```python
from build123d import *

# Parameters (mm, degrees)
SKETCH1_W           = 30.30738701
SKETCH1_H           = 30.002560534
BOSS_EXTRUDE1_DEPTH = 10
SKETCH2_R           = 9.6
SKETCH2_R_2         = 9.55
CUT_EXTRUDE1_DEPTH  = 7
SKETCH3_R           = 4
CUT_EXTRUDE2_DEPTH  = 10
SKETCH4_R           = 2
CUT_EXTRUDE3_DEPTH  = 10
CIRPATTERN1_COUNT   = 4


with BuildPart() as part:
    # Sketch1 → Boss-Extrude1 (new body)
    with BuildSketch(Plane(origin=(0, 0, 0), x_dir=(1, 0, 0), z_dir=(0, 1, 0))):
        Rectangle(SKETCH1_W, SKETCH1_H)
    extrude(amount=BOSS_EXTRUDE1_DEPTH)

    # Sketch2 → Cut-Extrude1 (cut)
    with BuildSketch(Plane(origin=(0, 10, 0), x_dir=(1, 0, 0), z_dir=(0, 1, 0))):
        Circle(SKETCH2_R)
        Circle(SKETCH2_R_2, mode=Mode.SUBTRACT)
    extrude(amount=-CUT_EXTRUDE1_DEPTH, mode=Mode.SUBTRACT)

    # Sketch3 → Cut-Extrude2 (cut)
    with BuildSketch(Plane(origin=(0, 10, 0), x_dir=(1, 0, 0), z_dir=(0, 1, 0))):
        Circle(SKETCH3_R)
    extrude(amount=-CUT_EXTRUDE2_DEPTH, mode=Mode.SUBTRACT)

    # Sketch4 → Cut-Extrude3 (cut)
    with BuildSketch(Plane(origin=(0, 10, 0), x_dir=(1, 0, 0), z_dir=(0, 1, 0))):
        with Locations((10.792349727, 10.987509758)):
            Circle(SKETCH4_R)
    cut_extrude3 = extrude(amount=-CUT_EXTRUDE3_DEPTH, mode=Mode.SUBTRACT)

    # CirPattern1: Cut-Extrude3 ×4 about axis
    cirpattern1_axis = Axis((0, 0, 0), (0, 1, 0))
    for i in range(1, CIRPATTERN1_COUNT):
        add(cut_extrude3.rotate(cirpattern1_axis, i * 360 / CIRPATTERN1_COUNT), mode=Mode.SUBTRACT)


solid = part.part
```
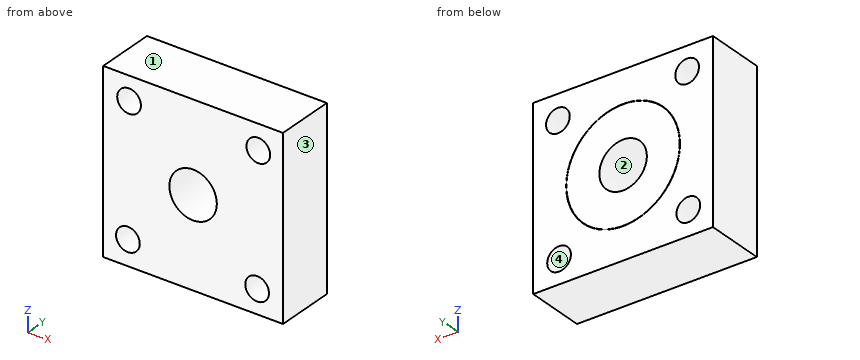
Read the model definition and answer for the solid it produces. Units are mm, in the model's axes. Face numbers are marked on the shaded views. Give positions to 0.01 mm unless a question says otherwise; leave off trailing zeros. Write each loop counter-clockwise with the first axis right and the second up, starting at its lowest first coordinate (ties: lowest second). Pieces come first, ordered by that corner, then holes. Notation, with made-up numbers: (54.5, -2) -> (108.5, -2) arc R15 cw to (108.5, 9) -> close; hole circle Ø1 at (46, 19). An arc over 180 degrees is marked (long way). Answer as a JSON object with one key per item and string values.
1) Section D-D on x = -12 is taken. Write down the section's boundary in (y, z).
Findings below:
{"outline": "(0, -15) -> (10, -15) -> (10, -12.52) -> (0, -12.52) -> close; (0, -9.07) -> (10, -9.07) -> (10, 9.39) -> (0, 9.39) -> close; (0, 12.58) -> (10, 12.58) -> (10, 15) -> (0, 15) -> close"}
2) Flat-ended cylindrical pins translate along their axes: pin 1 Ø5 at (x, z) = (0, 0) entering from +Y; pin 2 Ø5 at (x, z) = (3, -8) entering from -Y. Find the tip coordinate at first contact, or state that the pin passes through.
Findings below:
{"pin 1": "passes through", "pin 2": "stops at y = 0"}
3) Section C-C on y = 4.5 is taken. Write down the section's boundary in (x, z), then the cut area to 3 significant figures.
Findings below:
{"outline": "(-15.15, -15) -> (15.15, -15) -> (15.15, 15) -> (-15.15, 15) -> close; circle Ø19.1 at (0, 0); hole circle Ø4 at (-10.99, -10.79); hole circle Ø4 at (-10.79, 10.99); hole circle Ø19.2 at (0, 0); hole circle Ø8 at (0, 0); hole circle Ø4 at (10.79, -10.99); hole circle Ø4 at (10.99, 10.79)", "area": "806 mm^2"}
4) Straight lines are drawn through the part: probe 1 along Z at (x, y) = (-11, 8.5); probe 2 along Z at (x, y) = (10.5, 2.25); probe 3 along X at (y, z) = (1, 11.5). For each, find the intervals that lie inside material, in ascending order. Write a range as from..to.
Findings below:
{"probe 1": "z = -15..-12.79, -8.79..9, 12.98..15", "probe 2": "z = -15..-12.97, -9.01..8.85, 12.73..15", "probe 3": "x = -15.15..-12.73, -8.86..9.12, 12.86..15.15"}
5) Section A-A on z = 0 is taken. Write down the section's boundary in (x, y), then the cut area to 3 significant figures.
Findings below:
{"outline": "(-15.15, 0) -> (-4, 0) -> (-4, 10) -> (-9.55, 10) -> (-9.55, 3) -> (-9.6, 3) -> (-9.6, 10) -> (-15.15, 10) -> close; (4, 0) -> (15.15, 0) -> (15.15, 10) -> (9.6, 10) -> (9.6, 3) -> (9.55, 3) -> (9.55, 10) -> (4, 10) -> close", "area": "222 mm^2"}
6) Section B-B on x = 0 is taken. Write down the section's boundary in (y, z).
Findings below:
{"outline": "(0, -15) -> (10, -15) -> (10, -9.6) -> (3, -9.6) -> (3, -9.55) -> (10, -9.55) -> (10, -4) -> (0, -4) -> close; (0, 4) -> (10, 4) -> (10, 9.55) -> (3, 9.55) -> (3, 9.6) -> (10, 9.6) -> (10, 15) -> (0, 15) -> close"}
7) For a pull along X with two mould halves and no side action, classify the marked faces 1, 2, 3 and 4 as pulls with the +X half, pulls with the -X half, needs draft (parallel to the pull), parting line crosses it, or undercut.
Findings below:
{"face 1": "needs draft", "face 2": "undercut", "face 3": "pulls with the +X half", "face 4": "undercut"}
